Read the model definition and answer for the solid it produces. Units are mm, in the model's axes. Face numbers are marked on the shaded views. A direction names the side the tool comes from. Coordinates: 2 decimals unless noted, no trailing zeros. Write each loop counter-clockwise with the first axis right and the second up, starting at its lowest first coordinate (ties: lowest second). Pieces come first, ordered by that corner, then holes.
(1) Find the intervals of material crossed by probe 1 along Z at (x, y) = (12, 7.5); probe 2 along Z at (x, y) = (26.2, 4.5); probe 3 along X at (y, z) = (7.5, 8), in increasing order.
(2) Section A-A on x = 51.7 is taken. Write down the section's boundary in (y, z).
(3) Which of the six approach directions +Z, -Z, +X, -X, +Y, -Y give full straight-line access (tool end or side, diameter ignored) to the marked faces 5, 6, 7 and 8?
(4) Section D-D on z = -8 is taken. Write down the section's boundary in (x, y), then the cut area to 3 significant figures.
(5) Section B-B on x = -12 is taken. Write down the section's boundary in (y, z), then the cut area to 3 significant figures.
(6) The mould has two halves that part along Z. Classify the marked faces 1, 2, 3 and 4: +Z half, -Z half, draft (parallel to the pull), parting line (faces both ways), or undercut.
(7) Given pin 1 (5.5 mm diameter, centred on x = 41.2, z = 0, fed in from -Y); pin 2 (5 mm diameter, centred on y = 5.5, z = 11.5, fed in from +X); pin 3 (3 mm diameter, centred on y = 14, z = -5.5, fed in from -X); pin 4 (3 mm diameter, centred on y = 4.5, z = -25, fed in from +X), each flat-ended and moving along its own axis, determine where each tip first touches the part or whether it passes through.
(8) Section C-C on y = 10 is taken. Write down the section's boundary in (x, z), then the cut area to 3 significant figures.
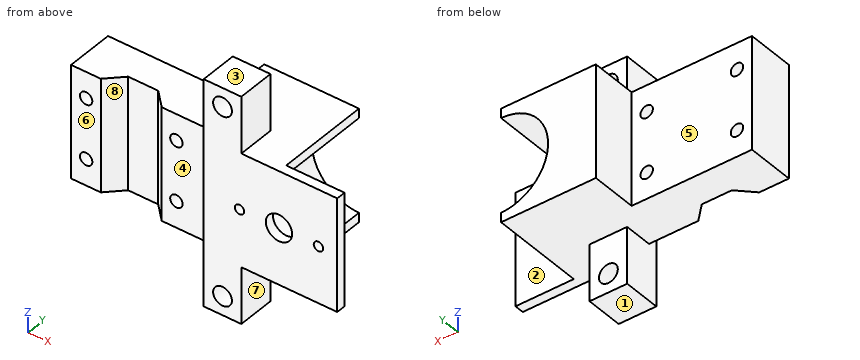
from build123d import *

# Parameters (mm, degrees)
BOSS_EXTRUDE1_DEPTH  = 15
SKETCH2_R            = 1.65
CUT_EXTRUDE1_DEPTH   = 12.7
SKETCH12_W           = 30
SKETCH12_H           = 25
BOSS_EXTRUDE9_DEPTH  = 25.2
CUT_EXTRUDE2_DEPTH   = 25
SKETCH14_W           = 35.5
SKETCH14_H           = 30
SKETCH14_R           = 3.5
SKETCH14_R_2         = 1.25
BOSS_EXTRUDE10_DEPTH = 2.5
SKETCH15_W           = 10
SKETCH15_H           = 15
SKETCH15_R           = 2.5
BOSS_EXTRUDE11_DEPTH = 10


with BuildPart() as part:
    # Sketch1 → Boss-Extrude1 (new body, symmetric)
    with BuildSketch(Plane.XY):
        Polygon((-4, 4.101219331), (4, 4.101219331), (8.101219331, 0), (16, 0), (16, 12.7), (-16, 12.7), (-16, 0), (-8.101219331, 0), align=None)
    extrude(amount=BOSS_EXTRUDE1_DEPTH, both=True)

    # Sketch2 → Cut-Extrude1 (cut)
    with BuildSketch(Plane(origin=(0, 12.7, 0), x_dir=(1, 0, 0), z_dir=(0, 1, 0))):
        with Locations((12, 8)):
            Circle(SKETCH2_R)
        with Locations((12, -8)):
            Circle(SKETCH2_R)
        with Locations((-12, -8)):
            Circle(SKETCH2_R)
        with Locations((-12, 8)):
            Circle(SKETCH2_R)
    extrude(amount=-CUT_EXTRUDE1_DEPTH, mode=Mode.SUBTRACT)

    # Sketch12 → Boss-Extrude9 (add)
    with BuildSketch(Plane(origin=(16, 0, 0), x_dir=(0, 0, -1), z_dir=(1, 0, 0))):
        with Locations((0, 12.5)):
            Rectangle(SKETCH12_W, SKETCH12_H)
    extrude(amount=BOSS_EXTRUDE9_DEPTH)

    # Sketch13 → Cut-Extrude2 (cut)
    with BuildSketch(Plane(origin=(0, 25, 0), x_dir=(1, 0, 0), z_dir=(0, 1, 0))):
        with BuildLine():
            Line((41.2, 12.5), (41.2, -12.5))
            ThreePointArc((41.2, -12.5), (28.7, 0), (41.2, 12.5))
        make_face()
    extrude(amount=-CUT_EXTRUDE2_DEPTH, mode=Mode.SUBTRACT)

    # Sketch14 → Boss-Extrude10 (add)
    with BuildSketch(Plane.XZ):
        with Locations((38.95, 0)):
            Rectangle(SKETCH14_W, SKETCH14_H)
        with Locations((41.2, 0)):
            Circle(SKETCH14_R, mode=Mode.SUBTRACT)
        with Locations((51.7, 0)):
            Circle(SKETCH14_R_2, mode=Mode.SUBTRACT)
        with Locations((30.7, 0)):
            Circle(SKETCH14_R_2, mode=Mode.SUBTRACT)
    extrude(amount=BOSS_EXTRUDE10_DEPTH)

    # Sketch15 → Boss-Extrude11 (add)
    with BuildSketch(Plane.XZ.offset(2.5)):
        with Locations((26.2, 22.5)):
            Rectangle(SKETCH15_W, SKETCH15_H)
        with Locations((26.2, 25)):
            Circle(SKETCH15_R, mode=Mode.SUBTRACT)
        with Locations((26.2, -22.5)):
            Rectangle(SKETCH15_W, SKETCH15_H)
        with Locations((26.2, -25)):
            Circle(SKETCH15_R, mode=Mode.SUBTRACT)
    extrude(amount=-BOSS_EXTRUDE11_DEPTH)


solid = part.part
Response:
1. probe 1: z = -15 to -9.65, -6.35 to 6.35, 9.65 to 15
1. probe 2: z = -30 to -27.5, -22.5 to 22.5, 27.5 to 30
1. probe 3: x = -16 to -13.65, -10.35 to 10.35, 13.65 to 31.6
2. outline: (-2.5, -15) - (0, -15) - (0, -1.25) - (-2.5, -1.25) - close; (-2.5, 1.25) - (0, 1.25) - (0, 15) - (-2.5, 15) - close
3. face 5: +Z, -Z, -X, +Y
3. face 6: +Z, -Z, -X, -Y
3. face 7: -Z, +X, +Y, -Y
3. face 8: +Z, -Z, -Y
4. outline: (-16, 0) - (-13.65, 0) - (-13.65, 12.7) - (-16, 12.7) - close; (-10.35, 0) - (-8.1, 0) - (-4, 4.1) - (4, 4.1) - (8.1, 0) - (10.35, 0) - (10.35, 12.7) - (-10.35, 12.7) - close; (13.65, 0) - (21.2, 0) - (21.2, -2.5) - (56.7, -2.5) - (56.7, 0) - (31.6, 0) - (31.6, 25) - (16, 25) - (16, 12.7) - (13.65, 12.7) - close
4. area: 752 mm2
5. outline: (0, -15) - (12.7, -15) - (12.7, -9.65) - (0, -9.65) - close; (0, -6.35) - (12.7, -6.35) - (12.7, 6.35) - (0, 6.35) - close; (0, 9.65) - (12.7, 9.65) - (12.7, 15) - (0, 15) - close
5. area: 297 mm2
6. face 1: -Z half
6. face 2: undercut
6. face 3: +Z half
6. face 4: draft
7. pin 1: passes through
7. pin 2: stops at x = 41.2
7. pin 3: stops at x = -16
7. pin 4: stops at x = 31.2
8. outline: (-16, -15) - (41.2, -15) - (41.2, -12.5) arc R12.5 cw to (41.2, 12.5) - (41.2, 15) - (-16, 15) - close; hole circle Ø3.3 at (-12, -8); hole circle Ø3.3 at (-12, 8); hole circle Ø3.3 at (12, -8); hole circle Ø3.3 at (12, 8)
8. area: 1,440 mm2
